```python
from build123d import *

# Parameters (mm, degrees)
SKETCH1_R           = 4.05
BOSS_EXTRUDE1_DEPTH = 6.7


with BuildPart() as part:
    # Sketch1 → Boss-Extrude1 (new body)
    with BuildSketch(Plane(origin=(0, 0, 0), x_dir=(1, 0, 0), z_dir=(0, 1, 0))):
        Polygon((3.167381974, -0.528493855), (3.167381974, 6.572914456), (-2.982618026, 10.123618611), (-9.132618026, 6.572914456), (-9.132618026, -0.528493855), (-2.982618026, -4.079198011), align=None)
        with Locations((-2.982618026, 3.0222103)):
            Circle(SKETCH1_R, mode=Mode.SUBTRACT)
    extrude(amount=BOSS_EXTRUDE1_DEPTH)


solid = part.part
```
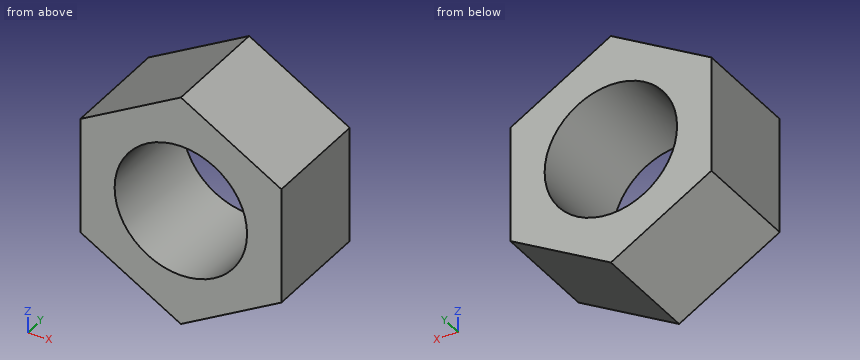
Work out the finished part from the listing and answer in its coordinate system (mm). Give positions to 0.01 mm unless a question says otherwise; leave off trailing zeros. Loops run counter-clockwise (first coordinate to the right, second up) from the corner with the lowest first, then second, coordinate; pieces in that order, holes last. Notation, with made-up numbers: (-38.5, 30) -> (19.5, 30) arc R12 ccw to (19.5, 36) -> close; hole circle Ø8 at (58, 77.25). An arc over 180 degrees is marked (long way). One line per question, with ' | ' between items. Start each with the question number.
1) Section A-A, the plane x = -1 is taken. Determine the outline of the cut face in (y, z).
2) Section D-D, the plane z = -8.75 is taken. Determine the outline of the cut face in (x, y).
3) Each of these flat-tipped pins is pushed along its axis until it touches: pin 1 (1 mm diameter, centred on x = 0, y = 5.5, fed in from +Z); pin 2 (3 mm diameter, centred on y = 4.5, z = -8.5, fed in from +X); pin 3 (1 mm diameter, centred on y = 5, z = 2, fed in from -X). Where does it stop, or does it pass through?
4) Section C-C, the plane y = 5.75 is taken. Determine the outline of the cut face in (x, z), then the cut area to 3 significant figures.
5) Section B-B, the plane z = -3.25 is taken. Determine the outline of the cut face in (x, y), then the cut area to 3 significant figures.
6) Straight lines are drawn through the part: L1, parallel to Z at x = -5.5, y = 6; L2, parallel to Z at x = -2, y = 4.5; L3, parallel to X at y = 2.25, z = -0.5. For each, find the intervals that lie inside material, in ascending order.
Resolved:
1) outline: (0, -8.98) -> (6.7, -8.98) -> (6.7, -6.55) -> (0, -6.55) -> close; (0, 0.51) -> (6.7, 0.51) -> (6.7, 2.93) -> (0, 2.93) -> close
2) outline: (-5.36, 0) -> (-0.6, 0) -> (-0.6, 6.7) -> (-5.36, 6.7) -> close
3) pin 1: z = 2.65 | pin 2: x = 2.43 | pin 3: x = -7.45
4) outline: (-9.13, -6.57) -> (-2.98, -10.12) -> (3.17, -6.57) -> (3.17, 0.53) -> (-2.98, 4.08) -> (-9.13, 0.53) -> close; hole circle Ø8.1 at (-2.98, -3.02) | area: 79.5 mm2
5) outline: (-9.13, 0) -> (-7.03, 0) -> (-7.03, 6.7) -> (-9.13, 6.7) -> close; (1.06, 0) -> (3.17, 0) -> (3.17, 6.7) -> (1.06, 6.7) -> close | area: 28.2 mm2
6) L1: -8.67 to -6.19, 0.15 to 2.63 | L2: -9.56 to -6.95, 0.91 to 3.51 | L3: -9.13 to -6.15, 0.19 to 3.17
